Read the model definition and answer for the solid it produces. Units are mm, in the model's axes. A direction names the side the tool comes from. Coordinates: 2 decimals unless noted, no trailing zeros. Write each loop counter-clockwise with the first axis right and the second up, starting at its lowest first coordinate (ties: lowest second). Pieces come first, ordered by that corner, then holes. Notation, with made-up numbers: (12.25, -12) -> (27.25, -12) arc R31 ccw to (27.25, 14) -> close; hole circle Ø9 at (-31.75, 28). An arc over 180 degrees is marked (long way). Answer in a Markdown table with one row per item. Add a question column.
Item 1: Section D-D on x = 0 is taken. Write down the section's boundary in (y, z), then the cut area to 3 significant figures.
Item 2: Section C-C on y = 0 is taken. Count the separate pieces of the cut face and the enclosed holes in it, then the cut area to 3 significant figures.
Item 3: Section B-B on y = -61.5 is taken. Write down the section's boundary in (x, z).
Item 4: Which of the six approach directions +Z, -Z, +X, -X, +Y, -Y give full straight-line access (tool end or side, diameter ignored) to faces 5 (the face through (77.5, -2.5, -10)), 6 (the face through (40, -60, -93)), 7 (the face through (-27, -23, -30))?
Item 5: Straight lines are drawn through the part: line 1 (Y direction, x = 0, z = -7.75); line 2 (Y direction, x = -80, z = -14.5); line 3 (Z direction, x = -40.5, y = -10.5). For each, find the intervals that lie inside material, in ascending order. Write a range as from..to.
Item 6: Given pin 1 Ø8.5 at (x, y) = (-80, 0) entering from +Z; pin 2 Ø2 at (x, z) = (19.5, -124.5) entering from +Y (3 decimals); pin 3 Ø24 at (x, y) = (-26, -18) entering from -Z; pin 4 Ø6 at (x, y) = (-82, 2.5) entering from -Z, each flat-ended and moving along its own axis, determine where each tip first touches the part or whether it passes through.
Item 7: For a pull along Y with two mould halves and no side action, classify faces 1 (the face through (-74.256, 0.253, -15.07)), 2 (the face through (1, -40, -10)), 3 (the face through (28, -23, -30)), 4 (the face through (119.99, 0.88, -9.86)) as +Y half, -Y half, draft (parallel to the pull), parting line (faces both ways), or undercut.
Item 8: Section A-A on z = -184 is taken. Write down the section's boundary in (x, y).
```python
from build123d import *

# Parameters (mm, degrees)
EXTRUDE_1_DEPTH     = 20
SKETCH_4_R          = 32.5
CUT_EXTRUDE_4_DEPTH = 10
SKETCH_10_W         = 25
SKETCH_10_H         = 77.5
EXTRUDE_5_DEPTH     = 10
SKETCH_14_W         = 25
SKETCH_14_H         = 15
EXTRUDE_6_DEPTH     = 200
CUT_EXTRUDE_5_DEPTH = 161
SKETCH_16_R         = 3.25
CUT_EXTRUDE_6_DEPTH = 21
SKETCH_17_R         = 5.75
CUT_EXTRUDE_7_DEPTH = 10


with BuildPart() as part:
    # 스케치3 → 보스-돌출1 (new body)
    with BuildSketch(Plane.XY):
        with BuildLine():
            Line((-80, 40), (80, 40))
            ThreePointArc((80, 40), (120, 0), (80, -40))
            Line((80, -40), (-80, -40))
            ThreePointArc((-80, -40), (-120, 0), (-80, 40))
        make_face()
    extrude(amount=-EXTRUDE_1_DEPTH)

    # 스케치4 → 컷-돌출4 (cut)
    with BuildSketch(Plane.XY):
        Circle(SKETCH_4_R)
    extrude(amount=-CUT_EXTRUDE_4_DEPTH, mode=Mode.SUBTRACT)

    # 스케치10 → 보스-돌출5 (add)
    with BuildSketch(Plane(origin=(0, 0, -20), x_dir=(-1, 0, 0), z_dir=(0, 0, -1))):
        with Locations((-27.5, -31.25)):
            Rectangle(SKETCH_10_W, SKETCH_10_H)
        with Locations((27.5, -31.25)):
            Rectangle(SKETCH_10_W, SKETCH_10_H)
    extrude(amount=EXTRUDE_5_DEPTH)

    # 스케치14 → 보스-돌출6 (add)
    with BuildSketch(Plane(origin=(0, 0, -30), x_dir=(-1, 0, 0), z_dir=(0, 0, -1))):
        with Locations((-27.5, -62.5)):
            Rectangle(SKETCH_14_W, SKETCH_14_H)
        with Locations((27.5, -62.5)):
            Rectangle(SKETCH_14_W, SKETCH_14_H)
    extrude(amount=EXTRUDE_6_DEPTH)

    # 스케치15 → 컷-돌출5 (cut, through all)
    with BuildSketch(Plane(origin=(40, 0, 0), x_dir=(0, 0, -1), z_dir=(1, 0, 0))):
        Polygon((30, -55), (230, -65), (230, -55), align=None)
    extrude(amount=-CUT_EXTRUDE_5_DEPTH, mode=Mode.SUBTRACT)

    # 스케치16 → 컷-돌출6 (cut, through all)
    with BuildSketch(Plane(origin=(0, 0, -20), x_dir=(-1, 0, 0), z_dir=(0, 0, -1))):
        with Locations((-80, 0)):
            Circle(SKETCH_16_R)
        with Locations((80, 0)):
            Circle(SKETCH_16_R)
    extrude(amount=-CUT_EXTRUDE_6_DEPTH, mode=Mode.SUBTRACT)

    # 스케치17 → 컷-돌출7 (cut)
    with BuildSketch(Plane(origin=(0, 0, -20), x_dir=(-1, 0, 0), z_dir=(0, 0, -1))):
        with Locations((-80, 0)):
            Circle(SKETCH_17_R)
        with Locations((80, 0)):
            Circle(SKETCH_17_R)
    extrude(amount=-CUT_EXTRUDE_7_DEPTH, mode=Mode.SUBTRACT)


solid = part.part
```
Results below:
| question | item | result |
|---|---|---|
| 1 | outline | (-40, -20) -> (40, -20) -> (40, 0) -> (32.5, 0) -> (32.5, -10) -> (-32.5, -10) -> (-32.5, 0) -> (-40, 0) -> close |
| 1 | area | 950 mm2 |
| 2 | separate pieces | 3 |
| 2 | enclosed holes | 0 |
| 2 | area | 4,290 mm2 |
| 3 | outline | (-40, -160) -> (-15, -160) -> (-15, -20) -> (-40, -20) -> close; (15, -160) -> (40, -160) -> (40, -20) -> (15, -20) -> close |
| 4 | face 5 | -Z |
| 4 | face 6 | -Z, +X, +Y, -Y |
| 4 | face 7 | -Z, +X, -X, +Y |
| 5 | line 1 | y = -40..-32.5, 32.5..40 |
| 5 | line 2 | y = -40..-5.75, 5.75..40 |
| 5 | line 3 | z = -20..0 |
| 6 | pin 1 | stops at z = 0 |
| 6 | pin 2 | stops at y = -59.675 |
| 6 | pin 3 | stops at z = -30 |
| 6 | pin 4 | stops at z = -20 |
| 7 | face 1 | undercut |
| 7 | face 2 | -Y half |
| 7 | face 3 | draft |
| 7 | face 4 | parting line |
| 8 | outline | (-40, -70) -> (-15, -70) -> (-15, -62.7) -> (-40, -62.7) -> close; (15, -70) -> (40, -70) -> (40, -62.7) -> (15, -62.7) -> close |
